```python
from build123d import *

# Parameters (mm, degrees)
ESQUISSE1_R                  = 1.5
BOSS_EXTRU_1_DEPTH           = 5
ENL_V_MAT_EXTRU_1_DEPTH      = 21.155644371
ENL_V_MAT_EXTRU_1_DEPTH_BACK = 21.155644371
ESQUISSE2_W                  = 2
ESQUISSE2_H                  = 8
CONG_1_R                     = 2


with BuildPart() as part:
    # Esquisse1 → Boss.-Extru.1 (new, symmetric)
    with BuildSketch(Plane(origin=(0, 0, 0), x_dir=(0, 0, -1), z_dir=(1, 0, 0))):
        with BuildLine():
            Line((2.572380753, 1.543650628), (12.5, -15))
            Line((12.5, -15), (-12.5, -15))
            Line((-12.5, -15), (-2.572380753, 1.543650628))
            ThreePointArc((-2.572380753, 1.543650628), (0, 3), (2.572380753, 1.543650628))
        make_face()
        Circle(ESQUISSE1_R, mode=Mode.SUBTRACT)
    extrude(amount=BOSS_EXTRU_1_DEPTH, both=True)

    # Esquisse2 → Enlèv. mat.-Extru.1 (cut, two sides: drawn at the far end of the back side and taken through both)
    with BuildSketch(Plane.XY.offset(-ENL_V_MAT_EXTRU_1_DEPTH_BACK)):
        with Locations((0, -1)):
            Rectangle(ESQUISSE2_W, ESQUISSE2_H)
    extrude(amount=ENL_V_MAT_EXTRU_1_DEPTH + ENL_V_MAT_EXTRU_1_DEPTH_BACK, mode=Mode.SUBTRACT)

    # Congé1
    cong_1_edges = [part.edges().sort_by_distance(p)[0] for p in [
        (0, -15, -12.5),
        (0, -15, 12.5),
    ]]
    fillet(cong_1_edges, radius=CONG_1_R)


solid = part.part
```
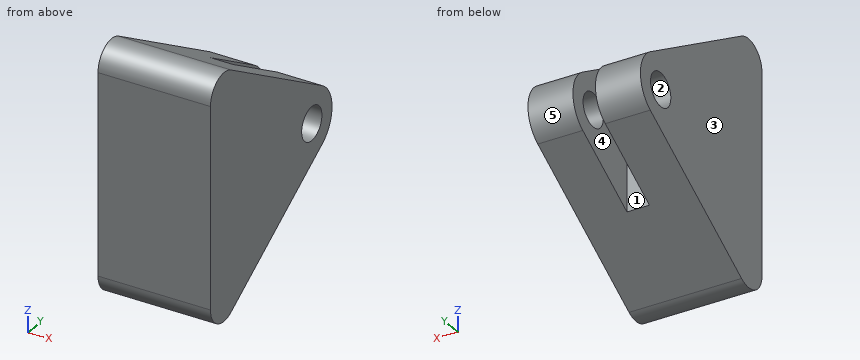
Here's how the part is built. I have some questions about the finished solid (model axes, mm). Face numbers are marked on the shaded views. A direction names the side the tool comes from. Give positions to 0.01 mm unless a question says otherwise; leave off trailing zeros. Loops run counter-clockwise (first coordinate to the right, second up) from the corner with the lowest first, then second, coordinate; pieces in that order, holes last. Notation, with made-up numbers: M 27,1 L 85,1 A19 cw 85,33 Z; hole C 35,-25 d7. An arc over 180 degrees is marked long. Use one line per item in the form item = value. Start each with the question number.
Q1. Will these pins go through, and if not, where does the flat tip stop? pin 1 Ø1 at (x, z) = (3.5, -1.5) entering from +Y; pin 2 Ø1.5 at (x, y) = (0, -12.5) entering from +Z; pin 3 Ø1.5 at (x, y) = (3.5, -1) entering from +Z; pin 4 Ø3 at (x, y) = (-1.5, -11) entering from -Z.
Q2. If we section it at D-D (y = -2): Write out the boundary of the cut face in (x, z), then the cut area to 3 significant figures.
Q3. Thinking about a two-plate mould opening in X: for the marked faces 3, 4 and 5, which applies, +X half, -X half, draft (parallel to the pull), parting line (faces both ways), or undercut?
Q4. Which directions (+Z, -Z, +X, -X, +Y, -Y) give clear straight access to the entire face, cutting with the end or side of a thin tool? Please do the marked faces 1 and 2.
Q5. If we section it at C-C (y = 0): Write out the boundary of the cut face in (x, z), then the cut area to 3 significant figures.
Q6. I need wall thicknesses on line 1 along Y through (x, z) = (3.55, 0); line 2 along Y through (x, z) = (3.75, -1.25); line 3 along X through (y, z) = (-2.75, -1.75). Which ranges of each line are inside material? Lowest first, please.
Q7. If we section it at A-A (z = 0): Write out the boundary of the cut face in (x, y).
Q8. If we section it at B-B (x = -2.25): Write out the boundary of the cut face in (y, z).
Taken from the geometry:
q1.pin_1 = 2.83
q1.pin_2 = 10.97
q1.pin_3 = 4.55
q1.pin_4 = -10.9
q2.outline = M -5,-4.7 L -1,-4.7 L -1,4.7 L -5,4.7 Z; M 1,-4.7 L 5,-4.7 L 5,4.7 L 1,4.7 Z
q2.area = 75.2 mm^2
q3.face_3 = -X half
q3.face_4 = undercut
q3.face_5 = draft
q4.face_1 = +Z, -Z, +Y
q4.face_2 = +X, -X
q5.outline = M -5,-3.5 L -1,-3.5 L -1,-1.5 L -5,-1.5 Z; M -5,1.5 L -1,1.5 L -1,3.5 L -5,3.5 Z; M 1,-3.5 L 5,-3.5 L 5,-1.5 L 1,-1.5 Z; M 1,1.5 L 5,1.5 L 5,3.5 L 1,3.5 Z
q5.area = 32.0 mm^2
q6.line_1 = -15 to -1.5, 1.5 to 3
q6.line_2 = -15 to -0.83, 0.83 to 2.73
q6.line_3 = -5 to -1, 1 to 5
q7.outline = M -5,-15 L 5,-15 L 5,-1.5 L 1,-1.5 L 1,-5 L -1,-5 L -1,-1.5 L -5,-1.5 Z; M -5,1.5 L -1,1.5 L -1,3 L -5,3 Z; M 1,1.5 L 5,1.5 L 5,3 L 1,3 Z
q8.outline = M -15,-8.97 A2 ccw -11.97,-10.68 L 1.54,-2.57 A3 ccw 1.54,2.57 L -11.97,10.68 A2 ccw -15,8.97 Z; hole C 0,0 d3
